Geometry: final body of the model. Coordinates: model frame, mm. A direction names the side the tool comes from. Give positions to 0.01 mm unless a question says otherwise; leave off trailing zeros. Answer as a JSON object with one key per item and string values. Group by question number.
(1) Material intervals for probe 1 along Y at (x, z) = (-90, 3.45); probe 2 along Y at (x, z) = (-159, 0.35); probe 3 along Y at (x, z) = (148.5, 2.75), sorted ascending.
(2) Set-up query: faces 4 (the face through (-98, -35, 2)), 5 (the face through (182.15, -26.99, 2.54)). Return all of +Z, -Z, +X, -X, +Y, -Y with unobstructed straight access to the full face (end or side cutting, diameter ignored); none if empty.
(3) Section query A-A on z = 3.8. State how many separate pieces and enclosed holes the cut face has, plus the area to 3 significant figures.
(4) Draft query along X for faces 1 (the face through (64, -35, 2)), 2 (the face through (-3, -5, 0)), 3 (the face through (152, -35, 2)). Return one class per face: +X half, -X half, draft (parallel to the pull), parting line (faces both ways), or undercut.
(5) Contact query for flat-ended pins moving along their axis: pin 1 Ø1.5 at (x, z) = (164, 1.5) entering from -Y; pin 2 Ø4 at (x, y) = (-90, 0) entering from -Z; pin 3 Ø2 at (x, z) = (105, 3.5) entering from -Y. Output: stop coordinate, or through.
from build123d import *

# Parameters (mm, degrees)
SKETCH1_R           = 1.25
BOSS_EXTRUDE1_DEPTH = 5
FILLET1_R           = 5
FILLET2_R           = 10


with BuildPart() as part:
    # Sketch1 → Boss-Extrude1 (new body)
    with BuildSketch(Plane.XY):
        Polygon((-185, -30), (-157, -30), (-147, -40), (-123, -40), (-113, -30), (-103, -30), (-93, -40), (-69, -40), (-59, -30), (-49, -30), (-39, -40), (-15, -40), (-5, -30), (5, -30), (15, -40), (39, -40), (49, -30), (59, -30), (69, -40), (93, -40), (103, -30), (113, -30), (123, -40), (147, -40), (157, -30), (185, -30), (185, 30), (-185, 30), align=None)
        with Locations((-90, 0)):
            Circle(SKETCH1_R, mode=Mode.SUBTRACT)
        with Locations(Location((90, 0, 0), (0, 0, 180))):
            Circle(SKETCH1_R, mode=Mode.SUBTRACT)
    extrude(amount=BOSS_EXTRUDE1_DEPTH)

    # Fillet1
    fillet1_edges = [part.edges().sort_by_distance(p)[0] for p in [
        (157, -30, 2.5),
        (147, -40, 2.5),
        (123, -40, 2.5),
        (113, -30, 2.5),
        (103, -30, 2.5),
        (93, -40, 2.5),
        (69, -40, 2.5),
        (59, -30, 2.5),
        (49, -30, 2.5),
        (39, -40, 2.5),
        (15, -40, 2.5),
        (5, -30, 2.5),
        (-5, -30, 2.5),
        (-15, -40, 2.5),
        (-39, -40, 2.5),
        (-49, -30, 2.5),
        (-59, -30, 2.5),
        (-69, -40, 2.5),
        (-93, -40, 2.5),
        (-103, -30, 2.5),
        (-113, -30, 2.5),
        (-123, -40, 2.5),
        (-147, -40, 2.5),
        (-157, -30, 2.5),
    ]]
    fillet(fillet1_edges, radius=FILLET1_R)

    # Fillet2
    fillet2_edges = [part.edges().sort_by_distance(p)[0] for p in [
        (185, -30, 2.5),
        (-185, -30, 2.5),
    ]]
    fillet(fillet2_edges, radius=FILLET2_R)


solid = part.part
Answer list:
{
 "1": {"probe 1": "-40 to -1.25, 1.25 to 30", "probe 2": "-30 to 30", "probe 3": "-38.5 to 30"},
 "2": {"face 4": "+Z, -Z, -Y", "face 5": "+Z, -Z, +X, -Y"},
 "3": {"separate pieces": "1", "enclosed holes": "2", "area": "24,200 mm2"},
 "4": {"face 1": "undercut", "face 2": "draft", "face 3": "+X half"},
 "5": {"pin 1": "y = -30", "pin 2": "z = 0", "pin 3": "y = -30.12"}
}
